Could you check a few things on this model? Use its own coordinates, in mm. Round coordinates to 2 decimals unless told otherwise and drop trailing zeros. Write each loop counter-clockwise with the first axis right and the second up, starting at its lowest first coordinate (ties: lowest second). Pieces come first, ordered by that corner, then holes. Notation, with made-up numbers: M 84.25,22.5 L 88.25,22.5 A13 ccw 88.25,30.5 Z; hole C -14.75,-3 d5. An arc over 180 degrees is marked long. One line per item, written item: value. Start each with the question number.
(1) If I drill on L1, parallel to Y at x = 55.5, z = 1.1; L2, parallel to Y at x = 15.38, z = 1.85 (3 decimals); L3, parallel to Y at x = 43, z = 2.2, over which ranges is the centre line in solid material (lowest first)?
(2) I want a section at D-D on x = 55.5. Please give me the cut outline in (y, z), and give its area (3 significant figures).
(3) Thinking about a two-plate mould opening in Y: for faces 1 (the face through (33, 32, 4)), 2 (the face through (29, 30.57, 2.03)), 3 (the face through (42, 44, 2)), which applies, released by +Y, released by -Y, zero draft, split by the parting line, or undercut?
(4) I want a section at C-C on z = 3.1. Please give me the cut outline in (x, y) (3 decimals), and give its area (3 significant figures).
(5) I want a section at B-B on y = 25. Please give me the cut outline in (x, z), and give its area (3 significant figures).
(6) I want a section at A-A on x = 46. Please give me the cut outline in (y, z), and give its area (3 significant figures).
```python
from build123d import *

# Parameters (mm, degrees)
SKETCH1_W             = 86
SKETCH1_H             = 44
BOSS_EXTRUDE1_DEPTH   = 4
SKETCH2_R             = 14
CUT_EXTRUDE1_DEPTH    = 4
SKETCH3_R             = 1.5
CUT_EXTRUDE3_DEPTH    = 4
F_1_0MM_DOWEL_HOLE1_D = 1.75


with BuildPart() as part:
    # Sketch1 → Boss-Extrude1 (new body)
    with BuildSketch(Plane.XY):
        with Locations((43, 22)):
            Rectangle(SKETCH1_W, SKETCH1_H)
    extrude(amount=BOSS_EXTRUDE1_DEPTH)

    # Sketch2 → Cut-Extrude1 (cut)
    with BuildSketch(Plane.XY.offset(4)):
        with Locations((43, 18)):
            Circle(SKETCH2_R)
    extrude(amount=-CUT_EXTRUDE1_DEPTH, mode=Mode.SUBTRACT)

    # Sketch3 → Cut-Extrude3 (cut)
    with BuildSketch(Plane.XY.offset(4)):
        with Locations((30.5, 30.5)):
            Circle(SKETCH3_R)
        with Locations((55.5, 30.5)):
            Circle(SKETCH3_R)
        with Locations((55.5, 5.5)):
            Circle(SKETCH3_R)
        with Locations((30.5, 5.5)):
            Circle(SKETCH3_R)
    extrude(amount=-CUT_EXTRUDE3_DEPTH, mode=Mode.SUBTRACT)

    # Ø1.0mm Dowel Hole1 (through all)
    with Locations(Plane.XY.offset(4)):
        with Locations((15.38, 10.75), (21.38, 10.75)):
            Hole(F_1_0MM_DOWEL_HOLE1_D / 2)


solid = part.part
```
Found:
1. L1: y = 0 to 4, 7 to 11.7, 24.3 to 29, 32 to 44
1. L2: y = 0 to 9.875, 11.625 to 44
1. L3: y = 0 to 4, 32 to 44
2. outline: M 0,0 L 4,0 L 4,4 L 0,4 Z; M 7,0 L 11.7,0 L 11.7,4 L 7,4 Z; M 24.3,0 L 29,0 L 29,4 L 24.3,4 Z; M 32,0 L 44,0 L 44,4 L 32,4 Z
2. area: 102 mm²
3. face 1: zero draft
3. face 2: undercut
3. face 3: released by +Y
4. outline: M 0,0 L 86,0 L 86,44 L 0,44 Z; hole C 15.38,10.75 d1.75; hole C 21.38,10.75 d1.75; hole C 30.5,5.5 d3; hole C 43,18 d28; hole C 30.5,30.5 d3; hole C 55.5,5.5 d3; hole C 55.5,30.5 d3
4. area: 3,140 mm²
5. outline: M 0,0 L 30.88,0 L 30.88,4 L 0,4 Z; M 55.12,0 L 86,0 L 86,4 L 55.12,4 Z
5. area: 247 mm²
6. outline: M 0,0 L 4.33,0 L 4.33,4 L 0,4 Z; M 31.67,0 L 44,0 L 44,4 L 31.67,4 Z
6. area: 66.6 mm²
